Answer from the drawing. Dimensions are ordinates in mm from the lowest x, y and z of the part. Round coordinates to 2 decimals unless told otherwise and drop trailing zeros. Order: outer loops, then holes, each group sorted by start corner. A loop starts at its lowest first (then second) coordinate and runs counter-clockwise, first axis right, second up. Notation, with made-up numbers: (6, 74) -> (12, 74) arc R5 cw to (12, 82) -> close; hole circle Ø7 at (42.5, 50). An arc over 180 degrees is marked (long way). Use a Markdown table: item, result. Add a question column.
1. The mould has two halves that part along Z. Classify the marked faces 1, 2 and 3: +Z half, -Z half, draft (parallel to the pull), parting line (faces both ways), or undercut.
2. Section A-A, the plane z = 1.5 is taken. Give the vertices of the cut face in (x, y) (1 decimal).
3. Given pin 1 (3.5 mm diameter, centred on x = 11.09, z = 4.96, fed in from -Y); pin 2 (1 mm diameter, centred on y = 6.5, z = 1.5, fed in from -X); pin 3 (5 mm diameter, centred on y = 2.5, z = 4, fed in from -X) (1 decimal); pin 4 (5 mm diameter, centred on y = 10, z = 3.5, fed in from +X), each flat-ended and moving along its own axis, determine where each tip first touches the part or whether it passes through.
4. Section C-C, the plane x = 9.75 is taken. Give the number of separate pieces and of enclosed holes in the cut face.
5. Section B-B, the plane z = 3.75 is taken. Give the vertices of the cut face in (x, y) (1 decimal), then the cut area to 3 significant figures.
6. Consider L1, parallel to X at y = 11, z = 6.25 (1 decimal); L2, parallel to X at y = 6.5, z = 3; L3, parallel to Y at x = 7, z = 7 (1 decimal). Determine where each line is inside the solid, lowest interval first. Write a range as [from, to].
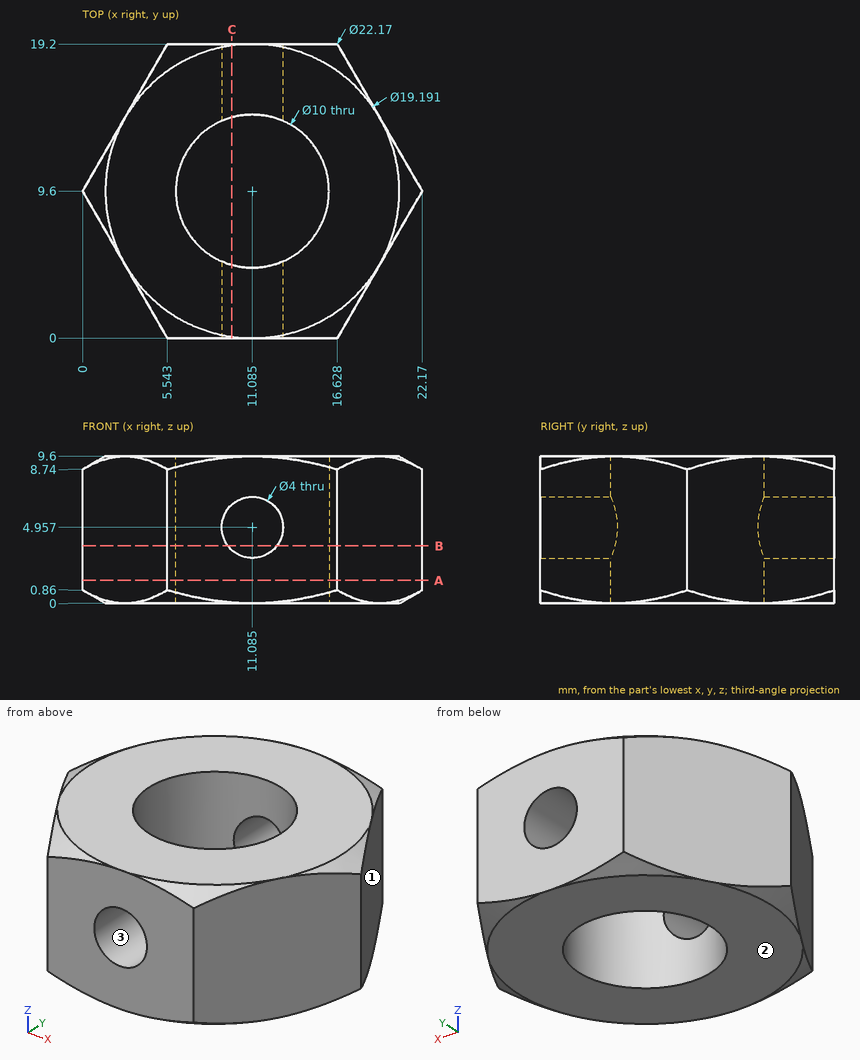
Verdict:
| question | item | result |
|---|---|---|
| 1 | face 1 | draft |
| 1 | face 2 | -Z half |
| 1 | face 3 | undercut |
| 2 | outline | (0, 9.6) -> (5.5, 0) -> (16.6, 0) -> (22.2, 9.6) -> (16.6, 19.2) -> (5.5, 19.2) -> close; hole circle Ø10 at (11.1, 9.6) |
| 3 | pin 1 | passes through |
| 3 | pin 2 | stops at x = 1.5 |
| 3 | pin 3 | stops at x = 2.7 |
| 3 | pin 4 | stops at x = 22.17 |
| 4 | separate pieces | 4 |
| 4 | enclosed holes | 0 |
| 5 | outline | (0, 9.6) -> (5.5, 0) -> (9.5, 0) -> (9.5, 4.9) arc R5 cw to (9.5, 14.3) -> (9.5, 19.2) -> (5.5, 19.2) -> close; (12.7, 0) -> (16.6, 0) -> (22.2, 9.6) -> (16.6, 19.2) -> (12.7, 19.2) -> (12.7, 14.3) arc R5 cw to (12.7, 4.9) -> close |
| 5 | area | 211 mm2 |
| 6 | L1 | x = [0.8, 6.3], [15.9, 21.4] |
| 6 | L2 | x = [1.79, 7.16], [15.01, 20.38] |
| 6 | L3 | y = [0, 6.7], [12.5, 19.2] |
